Geometry: final body of the model. Coordinates: model frame, mm. A direction names the side the tool comes from. Give positions to 0.01 mm unless a question says otherwise; leave off trailing zeros. Write each loop counter-clockwise with the first axis right and the second up, starting at its lowest first coordinate (ties: lowest second). Pieces come first, ordered by that corner, then holes.
from build123d import *

# Parameters (mm, degrees)
F0_R     = 19.05
F0_R_2   = 14.351381
F1_DEPTH = 25.4
F2_R     = 14.368686
F3_DEPTH = 7.62
F4_R     = 2.715155
F4_R_2   = 3.256151
F4_R_3   = 3.059417
F4_R_4   = 2.892412
F5_DEPTH = 17.781


with BuildPart() as f1:
    # F0 (on Front) → F1 (new body)
    with BuildSketch(Plane.XZ):
        Circle(F0_R)
        Circle(F0_R_2, mode=Mode.SUBTRACT)
        Circle(F0_R_2)
    extrude(amount=F1_DEPTH)

    # F2 (on face) → F3 (cut)
    with BuildSketch(Plane.XZ.offset(25.4)):
        Circle(F2_R)
    extrude(amount=-F3_DEPTH, mode=Mode.SUBTRACT)

    # F4 (on face) → F5 (cut, through all)
    with BuildSketch(Plane.XZ.offset(17.78)):
        with Locations((-7.626853, -5.900018)):
            Circle(F4_R)
        with Locations((-7.626853, 6.187824)):
            Circle(F4_R_2)
        with Locations((5.612213, 6.763435)):
            Circle(F4_R_3)
        with Locations((5.324407, -5.900018)):
            Circle(F4_R_4)
    extrude(amount=-F5_DEPTH, mode=Mode.SUBTRACT)


solid = f1.part
Q1. Section C-C on x = -3. Output: boundary loops of the cut face in (y, z), plus the area to 3 significant figures.
Filled sheet:
outline: (-25.4, -18.81) - (0, -18.81) - (0, 18.81) - (-25.4, 18.81) - (-25.4, 14.05) - (-17.78, 14.05) - (-17.78, -14.05) - (-25.4, -14.05) - close
area: 742 mm2
Q2. Pull-direction query (X, two-part tool) for faces 3 (the cylindrical face through (7.024, -9.014, 4.049)), 4 (the cylindrical face through (-15.12, -12.52, -11.59)), 5 (the cylindrical face through (3.19, -9.01, -3.95)), 6 (the flat face through (-7, -25.4, 13)); classes: released by +X, released by -X, zero draft, split by the parting line, or undercut.
Filled sheet:
face 3: undercut
face 4: split by the parting line
face 5: undercut
face 6: zero draft
Q3. Section B-B on x = 3.5. Output: boundary loops of the cut face in (y, z), plus the area to 3 significant figures.
Filled sheet:
outline: (-25.4, -18.73) - (0, -18.73) - (0, -8.14) - (-17.78, -8.14) - (-17.78, -13.94) - (-25.4, -13.94) - close; (-25.4, 13.94) - (-17.78, 13.94) - (-17.78, 8.98) - (0, 8.98) - (0, 18.73) - (-25.4, 18.73) - close; (-17.78, -3.66) - (0, -3.66) - (0, 4.55) - (-17.78, 4.55) - close
area: 580 mm2
Q4. Pin query (flat end, axial travel): P1, Ø6.5, axis at x = 5.32, z = -5.9, coming from the -Y side; P2, Ø5, axis at x = 13, y = -15, coming from the -Z side; P3, Ø3, axis at y = -14, z = 5.5, coming from the +X side. Return the tip coordinate at first contact, or that it passes through.
Filled sheet:
P1: stops at y = -17.78
P2: stops at z = -15.9
P3: stops at x = 18.63
Q5. Ray query, line 1 along Z through (x, y) = (4, -9.25); line 2 along Z through (x, y) = (4.5, -11.75); line 3 along X through (y, z) = (-16.25, -5.5). Return the intervals inside material, ascending.
Filled sheet:
line 1: z = -18.63 to -8.47, -3.33 to 4.16, 9.36 to 18.63
line 2: z = -18.51 to -8.67, -3.13 to 3.91, 9.61 to 18.51
line 3: x = -18.24 to -10.31, -4.94 to 2.46, 8.19 to 18.24
Q6. Access query for faces 1 (the flat face through (0, 0, 0)), 2 (the cylindrical face through (13.705, -21.643, 4.316)). Directions: +Z, -Z, +X, -X, +Y, -Y. A direction counts if a zero-diameter tool reaches every point of the face in a straight line with its end or side. Return the directions, or none.
Filled sheet:
face 1: +Z, -Z, +X, -X, +Y
face 2: -Y
Q7. Section A-A on z = 0. Output: boundary loops of the cut face in (x, y).
Filled sheet:
outline: (-19.05, -25.4) - (-14.37, -25.4) - (-14.37, -17.78) - (14.37, -17.78) - (14.37, -25.4) - (19.05, -25.4) - (19.05, 0) - (-19.05, 0) - close
Q8. Section D-D on y = -13. Output: boundary loops of the cut face in (x, z), plus the area to 3 significant figures.
Filled sheet:
outline: circle Ø38.1 at (0, 0); hole circle Ø6.51 at (-7.63, 6.19); hole circle Ø5.43 at (-7.63, -5.9); hole circle Ø5.78 at (5.32, -5.9); hole circle Ø6.12 at (5.61, 6.76)
area: 1,030 mm2
